Check sheet for the modelled part. Datum: model origin and axes. Units: mm. A direction names the side the tool comes from. Round coordinates to 2 decimals unless told otherwise and drop trailing zeros. Loops run counter-clockwise (first coordinate to the right, second up) from the corner with the lowest first, then second, coordinate; pieces in that order, holes last. Notation, with made-up numbers: (-16.5, 3.25) -> (11.5, 3.25) arc R19 ccw to (11.5, 30.25) -> close; hole circle Ø2 at (60.25, 8.25). An arc over 180 degrees is marked (long way). Use one line per item in the form item = value. Start each with the question number.
(1) Sectioned sample at A-A (x = 4.75). Record the cut outline in (y, z), and give its area (3 significant figures).
(2) Set-up check for faces 1 (the flat face through (-3, -5, -24)), 2 (the flat face through (2.428, 0, -24)), 3 (the flat face through (0, 2.428, -24)), 4 (the flat face through (-5, -7.5, -24)), 5 (the flat face through (7.5, -5, -24)): record each of +Z, -Z, +X, -X, +Y, -Y from which the full face is reachable in a straight line by a thin tool's end or side.
(3) Go/stop test with flat-tipped pins: pin 1 (5 mm diameter, centred on y = 4, z = -41, fed in from +X); pin 2 (3 mm diameter, centred on y = 5.5, z = -46.5, fed in from -X); pin 3 (2 mm diameter, centred on x = 4.5, z = -14.5, fed in from -Y). Record where each tip stops, or that it passes through.
(4) Material ranges on probe 1 along X at (y, z) = (1.75, -13); probe 2 along Y at (x, z) = (-3.5, -37); probe 3 along X at (y, z) = (-2.75, 17), recorded low to high. Write a range as [from, to].
(5) Draft check along Y on faces 6 (the flat face through (-7.5, -4, -24)), 7 (the flat face through (0, -2.428, -24)), 8 (the flat face through (5, 3, -24)). Enter one of: released by +Y, released by -Y, zero draft, split by the parting line, or undercut.
from build123d import *

# Parameters (mm, degrees)
F1_DEPTH = 75
F2_W     = 15.6
F2_H     = 15.6
F3_DEPTH = 50


# Not quite as in the source:
# - ends of sketch curves that miss each other by under 0.0002 mm in the source are joined


with BuildPart() as f1:
    # F0 (on Top) → F1 (new body, symmetric)
    with BuildSketch(Plane.XY):
        Polygon((7.5, 1.5), (7.5, 7.5), (1.5, 7.5), (1.5, 6), (3, 6), (3, 3.5), (1.1461396934, 2.7563427575), (1.1461396934, 2.42764467), (-1.1461396934, 2.42764467), (-1.1461396934, 2.7563427575), (-3, 3.5), (-3, 6), (-1.5, 6), (-1.5, 7.5), (-7.5, 7.5), (-7.5, 1.5), (-6, 1.5), (-6, 3), (-3.5, 3), (-2.7563427575, 1.1461396934), (-2.42764467, 1.1461396934), (-2.42764467, -1.1461396934), (-2.7563427575, -1.1461396934), (-3.5, -3), (-6, -3), (-6, -1.5), (-7.5, -1.5), (-7.5, -7.5), (-1.5, -7.5), (-1.5, -6), (-3, -6), (-3, -3.5), (-1.1461396934, -2.7563427575), (-1.1461396934, -2.42764467), (1.1461396934, -2.42764467), (1.1461396934, -2.7563427575), (3, -3.5), (3, -6), (1.5, -6), (1.5, -7.5), (7.5, -7.5), (7.5, -1.5), (6, -1.5), (6, -3), (3.5, -3), (2.7563427575, -1.1461396934), (2.42764467, -1.1461396934), (2.42764467, 1.1461396934), (2.7563427575, 1.1461396934), (3.5, 3), (6, 3), (6, 1.5), align=None)
    extrude(amount=F1_DEPTH, both=True)

    # F2 (on face) → F3 (join)
    with BuildSketch(Plane.XY.offset(75)):
        Rectangle(F2_W, F2_H)
        Polygon((7.5, 7.5), (7.5, 1.5), (6, 1.5), (6, 3), (3.5, 3), (2.7563427575, 1.1461396934), (2.42764467, 1.1461396934), (2.42764467, -1.1461396934), (2.7563427575, -1.1461396934), (3.5, -3), (6, -3), (6, -1.5), (7.5, -1.5), (7.5, -7.5), (1.5, -7.5), (1.5, -6), (3, -6), (3, -3.5), (1.1461396934, -2.7563427575), (1.1461396934, -2.42764467), (-1.1461396934, -2.42764467), (-1.1461396934, -2.7563427575), (-3, -3.5), (-3, -6), (-1.5, -6), (-1.5, -7.5), (-7.5, -7.5), (-7.5, -1.5), (-6, -1.5), (-6, -3), (-3.5, -3), (-2.7563427575, -1.1461396934), (-2.42764467, -1.1461396934), (-2.42764467, 1.1461396934), (-2.7563427575, 1.1461396934), (-3.5, 3), (-6, 3), (-6, 1.5), (-7.5, 1.5), (-7.5, 7.5), (-1.5, 7.5), (-1.5, 6), (-3, 6), (-3, 3.5), (-1.1461396934, 2.7563427575), (-1.1461396934, 2.42764467), (1.1461396934, 2.42764467), (1.1461396934, 2.7563427575), (3, 3.5), (3, 6), (1.5, 6), (1.5, 7.5), align=None, mode=Mode.SUBTRACT)
    extrude(amount=-F3_DEPTH)


solid = f1.part
Checks:
q1.outline = (-7.8, 25) -> (-7.5, 25) -> (-7.5, -75) -> (-3, -75) -> (-3, 25) -> (3, 25) -> (3, -75) -> (7.5, -75) -> (7.5, 25) -> (7.8, 25) -> (7.8, 75) -> (-7.8, 75) -> close
q1.area = 1,680 mm2
q2.face_1 = -Z
q2.face_2 = -Z, +X
q2.face_3 = -Z, +Y
q2.face_4 = -Z, +X, -X, -Y
q2.face_5 = -Z, +X, +Y, -Y
q3.pin_1 = 7.5
q3.pin_2 = -7.5
q3.pin_3 = -7.5
q4.probe_1 = [-7.5, -6], [-3, 3], [6, 7.5]
q4.probe_2 = [-7.5, -3], [3, 7.5]
q4.probe_3 = [-7.5, -6], [-3.4, -1.15], [1.15, 3.4], [6, 7.5]
q5.face_6 = zero draft
q5.face_7 = released by -Y
q5.face_8 = undercut
